The listing builds one solid part. Answer for the finished solid, in the listing's coordinates (mm). Round coordinates to 2 decimals unless told otherwise and drop trailing zeros. Write each loop counter-clockwise with the first axis right and the second up, starting at its lowest first coordinate (ties: lowest second). Pieces come first, ordered by that corner, then holes. Notation, with made-up numbers: (-38, -12.5) - (10, -12.5) arc R29 cw to (10, 24.5) - close; hole circle Ø2 at (-34.75, 60.5). An arc over 180 degrees is marked (long way). Return JSON: item names as keys, results as strings. Group by question number.
(1) Section A-A, the plane y = -40.5 is taken. Write down the section's boundary in (x, z) (3 decimals), then the cut area to 3 significant figures.
(2) Each of these flat-tipped pins is pushed along its axis until it touches: pin 1 (7.5 mm diameter, centred on x = 806.45, y = -25.4, fed in from -Z); pin 2 (1.5 mm diameter, centred on y = -45.5, z = 13.5, fed in from -X); pin 3 (5 mm diameter, centred on y = -18, z = 5.5, fed in from +X); pin 4 (11 mm diameter, centred on x = 1606.55, y = -25.4, fed in from -Z) (3 decimals). Where does it stop, or does it pass through?
(3) Find the intervals of material crossed by line 1 along X through (y, z) = (-25.5, 2.25); line 2 along X through (y, z) = (-33, 1.5); line 3 along Y through (x, z) = (806.45, 12.5), in increasing order. Write a range as [from, to].
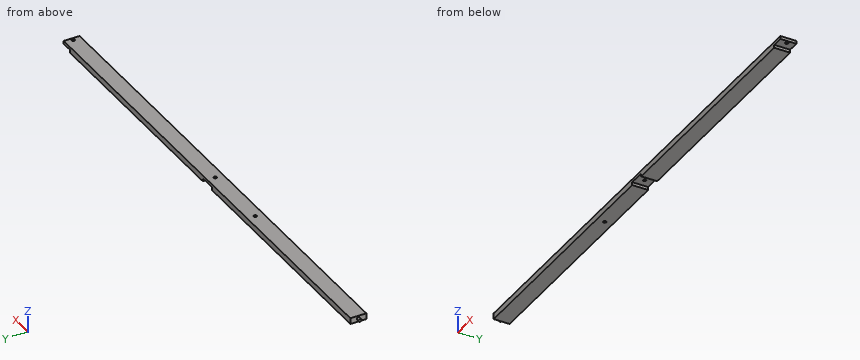
```python
from build123d import *

# Parameters (mm, degrees)
F1_DEPTH = 50.8
F3_R     = 4.7625
F4_DEPTH = 12.7
F5_R     = 4.7625
F6_DEPTH = 9.525


with BuildPart() as f1:
    # F0 (on Front) → F1 (new body)
    with BuildSketch(Plane.XZ):
        Polygon((1616.075, 9.525), (1616.075, 19.05), (0, 19.05), (0, 0), (781.05, 0), (781.05, 9.525), (831.85, 9.525), (831.85, 0), (1581.15, 0), (1581.15, 9.525), align=None)
    extrude(amount=F1_DEPTH)

    # F3 (on offset) → F4 (cut, symmetric)
    with BuildSketch(Plane.XY.offset(9.525)):
        with Locations((806.45, -25.4)):
            Circle(F3_R)
        with Locations((1606.55, -25.4)):
            Circle(F3_R)
        with Locations((581.025, -25.4)):
            Circle(F3_R)
    extrude(amount=F4_DEPTH, both=True, mode=Mode.SUBTRACT)

    # F5 (on Right) → F6 (join)
    with BuildSketch(Plane.YZ):
        with Locations((-25.4, 9.525)):
            Circle(F5_R)
    extrude(amount=-F6_DEPTH)


solid = f1.part
```
Working result:
{
 "1": {"outline": "(0, 0) - (781.05, 0) - (781.05, 9.525) - (831.85, 9.525) - (831.85, 0) - (1581.15, 0) - (1581.15, 9.525) - (1616.075, 9.525) - (1616.075, 19.05) - (0, 19.05) - close", "area": "30,000 mm^2"},
 "2": {"pin 1": "passes through", "pin 2": "stops at x = 0", "pin 3": "stops at x = 1581.15", "pin 4": "stops at z = 9.525"},
 "3": {"line 1": "x = [0, 576.26], [585.79, 781.05], [831.85, 1581.15]", "line 2": "x = [0, 781.05], [831.85, 1581.15]", "line 3": "y = [-50.8, -30.16], [-20.64, 0]"}
}
